Geometry check sheet. Reference: drawing and pictorial views, mm from the part's lowest x, y, z. Give positions to 0.01 mm unless a question says otherwise; leave off trailing zeros. Loops run counter-clockwise (first coordinate to the right, second up) from the corner with the lowest first, then second, coordinate; pieces in that order, holes last. Notation, with made-up numbers: (86, 51) - (123, 51) arc R26 cw to (123, 75) - close; hole circle Ø7 at (57, 12.5). An arc over 180 degrees is marked (long way). Put each result on its own line as item: value. Start each with the question number.
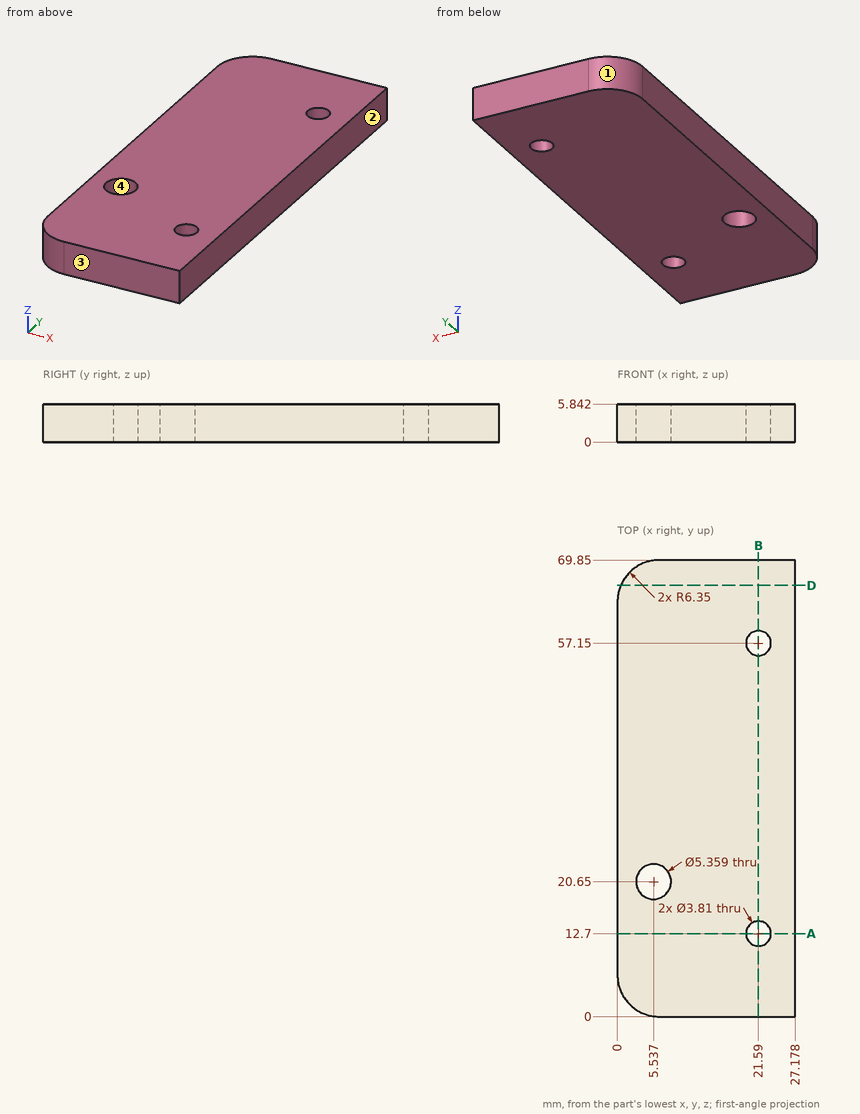
1) Draft check along X on the marked faces 1, 2, 3 and 4. Enter one of: pulls with the +X half, pulls with the -X half, needs draft (parallel to the pull), parting line crosses it, or undercut.
2) Scan lines: line 1 along X through (y, z) = (57.15, 4.45) (1 decimal); line 2 along Y through (x, z) = (4.25, 2.55); line 3 along X through (y, z) = (22, 1.2). Record each from-to range of solid material in increasing order. Write a range as from..to.
3) Depth check by flat-ended pin: P1, Ø2, axis at x = 5, z = 1, coming from the +Y side; P2, Ø4.5, axis at x = 5.54, y = 20.65, coming from the -Z side. Enter the tip coordinate at first touch or a pass-through.
4) Section check D-D, the plane y = 66. Enter the section's corners in (x, z), plus the area to 3 significant figures.
5) Section check A-A, the plane y = 12.7. Enter the section's corners in (x, z) (1 decimal).
6) Section check B-B, the plane x = 21.59. State how many separate pieces and enclosed holes the cut face has.
Results are:
1. face 1: pulls with the -X half
1. face 2: pulls with the +X half
1. face 3: needs draft
1. face 4: undercut
2. line 1: x = 0..19.7, 23.5..27.2
2. line 2: y = 0.36..18.3, 23..69.49
2. line 3: x = 0..3.22, 7.85..27.18
3. P1: stops at y = 69.84
3. P2: passes through
4. outline: (0.51, 0) - (27.18, 0) - (27.18, 5.84) - (0.51, 5.84) - close
4. area: 156 mm2
5. outline: (0, 0) - (19.7, 0) - (19.7, 5.8) - (0, 5.8) - close; (23.5, 0) - (27.2, 0) - (27.2, 5.8) - (23.5, 5.8) - close
6. separate pieces: 3
6. enclosed holes: 0
